Input: part model. Units: mm. Frame: model coordinates. A direction names the side the tool comes from. Coordinates: 2 decimals unless noted, no trailing zeros. Write each loop counter-clockwise with the first axis right and the second up, starting at its lowest first coordinate (ties: lowest second). Pieces come first, ordered by that corner, then holes. Notation, with made-up numbers: (-17, 71) -> (-12, 71) arc R23 ccw to (-12, 96) -> close; hole circle Ø2 at (77.25, -27.5). An arc over 180 degrees is marked (long way). Use one line per item in the form item = value. Start each with the question number.
(1) Cut plane B-B on z = -5.5. Return the cut outline in (x, y), plus the area to 3 significant figures.
(2) First-contact query: pin 1 (1.2 mm diameter, centred on x = 82.5, z = -6, fed in from +Y); pin 2 (5 mm diameter, centred on x = 95, y = -8.5, fed in from +Z); pin 3 (8 mm diameter, centred on x = 24, z = -18.5, fed in from -Y). Flat tips, straight axial feed; report the tip coordinate or a pass-through.
(3) Pull-direction query (X, two-part tool) for faces 3 (the face through (0, 0, -5)), 4 (the face through (119, -3, -5)), 5 (the face through (55, 1.924, -5)); classes: released by +X, released by -X, zero draft, split by the parting line, or undercut.
(4) Cut plane A-A on x = 13.5. Return the cut outline in (y, z), plus the area to 3 significant figures.
(5) Ray query, line 1 along X through (y, z) = (-4, -18); line 2 along X through (y, z) = (-4.25, -10); line 3 along X through (y, z) = (-0.5, 4.5). Return the intervals inside material, ascending.
(6) Set-up query: faces 1 (the face through (55, -13.076, -5)), 2 (the face through (87.472, -3.83, -19.734)). Return all of +Z, -Z, +X, -X, +Y, -Y with unobstructed straight access to the full face (end or side cutting, diameter ignored); none if empty.
```python
from build123d import *

# Parameters (mm, degrees)
SALIENTE_EXTRUIR1_DEPTH = 111
CROQUIS2_W              = 111
CROQUIS2_H              = 5
CORTAR_EXTRUIR1_DEPTH   = 5
CROQUIS3_W              = 111
CROQUIS3_H              = 5
CORTAR_EXTRUIR2_DEPTH   = 5
CROQUIS8_W              = 111
CROQUIS8_H              = 5
SALIENTE_EXTRUIR6_DEPTH = 5
CROQUIS9_W              = 111
CROQUIS9_H              = 5
SALIENTE_EXTRUIR7_DEPTH = 5
CROQUIS10_W             = 111
CROQUIS10_H             = 5
SALIENTE_EXTRUIR8_DEPTH = 5
CROQUIS11_W             = 111
CROQUIS11_H             = 5
SALIENTE_EXTRUIR9_DEPTH = 5
SALIENTE_EXTRUIR2_DEPTH = 8
SALIENTE_EXTRUIR3_DEPTH = 2
SALIENTE_EXTRUIR4_DEPTH = 8
SALIENTE_EXTRUIR5_DEPTH = 2
CROQUIS12_R             = 2
CORTAR_EXTRUIR3_DEPTH   = 16
CROQUIS13_R             = 4
CORTAR_EXTRUIR4_DEPTH   = 4
CROQUIS14_R             = 2
CORTAR_EXTRUIR5_DEPTH   = 16
CROQUIS15_R             = 4
CORTAR_EXTRUIR6_DEPTH   = 4


with BuildPart() as part:
    # Croquis1 → Saliente-Extruir1 (new body)
    with BuildSketch(Plane(origin=(0, 0, 0), x_dir=(0, 0, -1), z_dir=(1, 0, 0))):
        with BuildLine():
            Line((2.336042938, 2.185332004), (-2.204135338, 4.767752626))
            Line((-2.204135338, 4.767752626), (-7.148243501, -3.924530991))
            Line((-7.148243501, -3.924530991), (-2.608065225, -6.506951614))
            ThreePointArc((-2.608065225, -6.506951614), (0.256386453, -7.677264762), (3.32486457, -8.076211273))
            Line((3.32486457, -8.076211273), (7.253055883, -8.076211273))
            ThreePointArc((7.253055883, -8.076211273), (10.396202626, -7.657257363), (13.3198771, -6.429649364))
            Line((13.3198771, -6.429649364), (17.85154901, -3.774218091))
            Line((17.85154901, -3.774218091), (12.795864662, 4.853646985))
            Line((12.795864662, 4.853646985), (8.264192752, 2.198215712))
            ThreePointArc((8.264192752, 2.198215712), (7.776913673, 1.993614379), (7.253055883, 1.923788727))
            Line((7.253055883, 1.923788727), (3.32486457, 1.923788727))
            ThreePointArc((3.32486457, 1.923788727), (2.813451551, 1.990279812), (2.336042938, 2.185332004))
        make_face()
        with BuildLine():
            Line((-2.608065225, -6.506951614), (-7.148243501, -3.924530991))
            Line((-7.148243501, -3.924530991), (-9.620297582, -8.270672799))
            Line((-9.620297582, -8.270672799), (-5.080119306, -10.853093422))
            ThreePointArc((-5.080119306, -10.853093422), (-1.022146096, -12.511037048), (3.32486457, -13.076211273))
            Line((3.32486457, -13.076211273), (7.253055883, -13.076211273))
            ThreePointArc((7.253055883, -13.076211273), (11.705847103, -12.482693234), (15.847719275, -10.743581902))
            Line((15.847719275, -10.743581902), (20.379391184, -8.088150629))
            Line((20.379391184, -8.088150629), (17.85154901, -3.774218091))
            Line((17.85154901, -3.774218091), (13.3198771, -6.429649364))
            ThreePointArc((13.3198771, -6.429649364), (10.396202626, -7.657257363), (7.253055883, -8.076211273))
            Line((7.253055883, -8.076211273), (3.32486457, -8.076211273))
            ThreePointArc((3.32486457, -8.076211273), (0.256386453, -7.677264762), (-2.608065225, -6.506951614))
        make_face()
    extrude(amount=SALIENTE_EXTRUIR1_DEPTH)

    # Croquis2 → Cortar-Extruir1 (cut)
    with BuildSketch(Plane(origin=(0, 6.822115228, -11.642398074), x_dir=(1, 0, 0), z_dir=(0, 0.505568435, -0.862786508))):
        with Locations((55.5, 9.781524138)):
            Rectangle(CROQUIS2_W, CROQUIS2_H)
    extrude(amount=-CORTAR_EXTRUIR1_DEPTH, mode=Mode.SUBTRACT)

    # Croquis3 → Cortar-Extruir2 (cut)
    with BuildSketch(Plane(origin=(0, 2.112679425, 3.714321805), x_dir=(1, 0, 0), z_dir=(0, 0.494410816, 0.869228362))):
        with Locations((55.5, -4.445482547)):
            Rectangle(CROQUIS3_W, CROQUIS3_H)
    extrude(amount=-CORTAR_EXTRUIR2_DEPTH, mode=Mode.SUBTRACT)

    # Croquis8 → Saliente-Extruir6 (add)
    with BuildSketch(Plane(origin=(0, 2.112679425, 3.714321805), x_dir=(1, 0, 0), z_dir=(0, 0.494410816, 0.869228362))):
        with Locations((55.5, 0.554517453)):
            Rectangle(CROQUIS8_W, CROQUIS8_H)
    extrude(amount=SALIENTE_EXTRUIR6_DEPTH)

    # Croquis9 → Saliente-Extruir7 (add)
    with BuildSketch(Plane(origin=(0, 2.112679425, 3.714321805), x_dir=(1, 0, 0), z_dir=(0, 0.494410816, 0.869228362))):
        with Locations((55.5, -9.445482547)):
            Rectangle(CROQUIS9_W, CROQUIS9_H)
    extrude(amount=SALIENTE_EXTRUIR7_DEPTH)

    # Croquis10 → Saliente-Extruir8 (add)
    with BuildSketch(Plane(origin=(0, 6.822115228, -11.642398074), x_dir=(-1, 0, 0), z_dir=(0, 0.505568435, -0.862786508))):
        with Locations((-55.5, -4.781524138)):
            Rectangle(CROQUIS10_W, CROQUIS10_H)
    extrude(amount=SALIENTE_EXTRUIR8_DEPTH)

    # Croquis11 → Saliente-Extruir9 (add)
    with BuildSketch(Plane(origin=(0, 6.822115228, -11.642398074), x_dir=(-1, 0, 0), z_dir=(0, 0.505568435, -0.862786508))):
        with Locations((-55.5, -14.781524138)):
            Rectangle(CROQUIS11_W, CROQUIS11_H)
    extrude(amount=SALIENTE_EXTRUIR9_DEPTH)

    # Croquis4 → Saliente-Extruir2 (add)
    with BuildSketch(Plane.ZY):
        with BuildLine():
            Line((2.802101692, -6.396585072), (-13.537616472, -6.302060265))
            Line((-13.537616472, -6.302060265), (-22.165481548, -1.246375917))
            Line((-22.165481548, -1.246375917), (-24.693323722, -5.560308455))
            Line((-24.693323722, -5.560308455), (-15.847719275, -10.743581902))
            ThreePointArc((-15.847719275, -10.743581902), (-11.705847103, -12.482693234), (-7.253055883, -13.076211273))
            Line((-7.253055883, -13.076211273), (-3.32486457, -13.076211273))
            ThreePointArc((-3.32486457, -13.076211273), (1.022146096, -12.511037048), (5.080119306, -10.853093422))
            Line((5.080119306, -10.853093422), (13.96643939, -5.798618718))
            Line((13.96643939, -5.798618718), (11.494385309, -1.452476909))
            Line((11.494385309, -1.452476909), (2.802101692, -6.396585072))
        make_face()
    extrude(amount=SALIENTE_EXTRUIR2_DEPTH)

    # Croquis5 → Saliente-Extruir3 (add)
    with BuildSketch(Plane.ZY.offset(8)):
        with BuildLine():
            Line((-8.264192752, 2.198215712), (-17.1097972, 7.381489159))
            Line((-17.1097972, 7.381489159), (-22.165481548, -1.246375917))
            Line((-22.165481548, -1.246375917), (-13.537616472, -6.302060265))
            Line((-13.537616472, -6.302060265), (2.802101692, -6.396585072))
            Line((2.802101692, -6.396585072), (11.494385309, -1.452476909))
            Line((11.494385309, -1.452476909), (6.550277147, 7.239806708))
            Line((6.550277147, 7.239806708), (-2.336042938, 2.185332004))
            ThreePointArc((-2.336042938, 2.185332004), (-2.813451551, 1.990279812), (-3.32486457, 1.923788727))
            Line((-3.32486457, 1.923788727), (-7.253055883, 1.923788727))
            ThreePointArc((-7.253055883, 1.923788727), (-7.776913673, 1.993614379), (-8.264192752, 2.198215712))
        make_face()
    extrude(amount=-SALIENTE_EXTRUIR3_DEPTH)

    # Croquis6 → Saliente-Extruir4 (add)
    with BuildSketch(Plane(origin=(111, 0, 0), x_dir=(0, 0, -1), z_dir=(1, 0, 0))):
        with BuildLine():
            Line((13.537616472, -6.302060265), (-2.802101692, -6.396585072))
            Line((-2.802101692, -6.396585072), (-11.494385309, -1.452476909))
            Line((-11.494385309, -1.452476909), (-13.96643939, -5.798618718))
            Line((-13.96643939, -5.798618718), (-5.080119306, -10.853093422))
            ThreePointArc((-5.080119306, -10.853093422), (-1.022146096, -12.511037048), (3.32486457, -13.076211273))
            Line((3.32486457, -13.076211273), (7.253055883, -13.076211273))
            ThreePointArc((7.253055883, -13.076211273), (11.705847103, -12.482693234), (15.847719275, -10.743581902))
            Line((15.847719275, -10.743581902), (24.693323722, -5.560308455))
            Line((24.693323722, -5.560308455), (22.165481548, -1.246375917))
            Line((22.165481548, -1.246375917), (13.537616472, -6.302060265))
        make_face()
    extrude(amount=SALIENTE_EXTRUIR4_DEPTH)

    # Croquis7 → Saliente-Extruir5 (add)
    with BuildSketch(Plane(origin=(119, 0, 0), x_dir=(0, 0, -1), z_dir=(1, 0, 0))):
        with BuildLine():
            Line((22.165481548, -1.246375917), (17.1097972, 7.381489159))
            Line((17.1097972, 7.381489159), (8.264192752, 2.198215712))
            ThreePointArc((8.264192752, 2.198215712), (7.776913673, 1.993614379), (7.253055883, 1.923788727))
            Line((7.253055883, 1.923788727), (3.32486457, 1.923788727))
            ThreePointArc((3.32486457, 1.923788727), (2.813451551, 1.990279812), (2.336042938, 2.185332004))
            Line((2.336042938, 2.185332004), (-6.550277147, 7.239806708))
            Line((-6.550277147, 7.239806708), (-11.494385309, -1.452476909))
            Line((-11.494385309, -1.452476909), (-2.802101692, -6.396585072))
            Line((-2.802101692, -6.396585072), (13.537616472, -6.302060265))
            Line((13.537616472, -6.302060265), (22.165481548, -1.246375917))
        make_face()
    extrude(amount=-SALIENTE_EXTRUIR5_DEPTH)

    # Croquis12 → Cortar-Extruir3 (cut)
    with BuildSketch(Plane(origin=(0, -10.383352224, 5.905975776), x_dir=(-1, 0, 0), z_dir=(0, -0.869228362, 0.494410816))):
        with Locations((-23.25, -4.16151121)):
            Circle(CROQUIS12_R)
        with Locations((-54.5, -4.16151121)):
            Circle(CROQUIS12_R)
        with Locations((-85.75, -4.16151121)):
            Circle(CROQUIS12_R)
    extrude(amount=-CORTAR_EXTRUIR3_DEPTH, mode=Mode.SUBTRACT)

    # Croquis13 → Cortar-Extruir4 (cut)
    with BuildSketch(Plane(origin=(0, -10.383352224, 5.905975776), x_dir=(1, 0, 0), z_dir=(0, -0.869228362, 0.494410816))):
        with Locations((23.25, 4.16151121)):
            Circle(CROQUIS13_R)
        with Locations((54.5, 4.16151121)):
            Circle(CROQUIS13_R)
        with Locations((85.75, 4.16151121)):
            Circle(CROQUIS13_R)
    extrude(amount=-CORTAR_EXTRUIR4_DEPTH, mode=Mode.SUBTRACT)

    # Croquis14 → Cortar-Extruir5 (cut)
    with BuildSketch(Plane(origin=(0, -14.910265857, -8.73699311), x_dir=(-1, 0, 0), z_dir=(0, -0.862786508, -0.505568435))):
        with Locations((-23.25, 13.367766286)):
            Circle(CROQUIS14_R)
        with Locations((-54.5, 13.367766286)):
            Circle(CROQUIS14_R)
        with Locations((-85.75, 13.367766286)):
            Circle(CROQUIS14_R)
    extrude(amount=-CORTAR_EXTRUIR5_DEPTH, mode=Mode.SUBTRACT)

    # Croquis15 → Cortar-Extruir6 (cut)
    with BuildSketch(Plane(origin=(0, -14.910265857, -8.73699311), x_dir=(1, 0, 0), z_dir=(0, -0.862786508, -0.505568435))):
        with Locations((23.25, -13.367766286)):
            Circle(CROQUIS15_R)
        with Locations((54.5, -13.367766286)):
            Circle(CROQUIS15_R)
        with Locations((85.75, -13.367766286)):
            Circle(CROQUIS15_R)
    extrude(amount=-CORTAR_EXTRUIR6_DEPTH, mode=Mode.SUBTRACT)


solid = part.part
```
Values:
q1.outline = (-8, -13.08) -> (119, -13.08) -> (119, 1.92) -> (117, 1.92) -> (117, -6.35) -> (111, -6.35) -> (111, 1.92) -> (0, 1.92) -> (0, -6.35) -> (-6, -6.35) -> (-6, 1.92) -> (-8, 1.92) -> close
q1.area = 1,810 mm2
q2.pin_1 = 1.92
q2.pin_2 = 13.61
q2.pin_3 = -11.45
q3.face_3 = undercut
q3.face_4 = released by +X
q3.face_5 = zero draft
q4.outline = (-13.08, -7.25) arc R17 ccw to (-10.74, -15.85) -> (-5.56, -24.69) -> (-1.25, -22.17) -> (-6.3, -13.54) -> (-1.99, -11.01) -> (3.07, -19.64) -> (7.38, -17.11) -> (2.2, -8.26) arc R2 cw to (1.92, -7.25) -> (1.92, -3.32) arc R2 cw to (2.19, -2.34) -> (7.24, 6.55) -> (2.89, 9.02) -> (-2.05, 0.33) -> (-6.4, 2.8) -> (-1.45, 11.49) -> (-5.8, 13.97) -> (-10.85, 5.08) arc R17 ccw to (-13.08, -3.32) -> close
q4.area = 415 mm2
q5.line_1 = -8 to 21.25, 25.25 to 52.5, 56.5 to 83.75, 87.75 to 119
q5.line_2 = -8 to -6, 0 to 111, 117 to 119
q5.line_3 = -8 to -6, 117 to 119
q6.face_1 = +Z, -Z, +X, -X, -Y
q6.face_2 = none
